Build history of the part. All positions in model axes, mm. Give positions to 0.01 mm unless a question says otherwise; leave off trailing zeros. Write each loop counter-clockwise with the first axis right and the second up, starting at its lowest first coordinate (ties: lowest second). Pieces come first, ordered by that corner, then holes. Notation, with made-up numbers: (54, -36.5) -> (97, -36.5) arc R29 ccw to (97, -7.5) -> close; hole circle Ø3 at (89, 79.25). An arc over 180 degrees is marked (long way). Put each result on its own line as item: value.
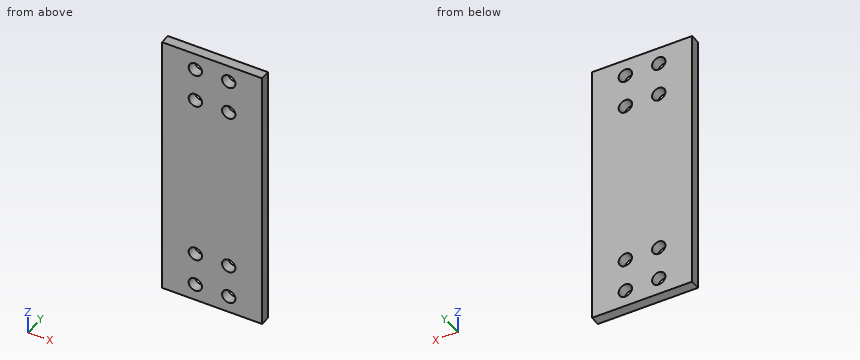
from build123d import *

# Parameters (mm, degrees)
SKETCH2_W           = 15
SKETCH2_H           = 40
SKETCH2_R           = 2
BOSS_EXTRUDE1_DEPTH = 3
MIRROR1_OUTLINE_R   = 2
MIRROR1_DEPTH       = 3


# Read off the part's stored shape, not the designer's step: Mirror1
with BuildPart() as part:
    # Sketch2 → Boss-Extrude1 (new body)
    with BuildSketch(Plane(origin=(0, 0, 0), x_dir=(1, 0, 0), z_dir=(0, 1, 0))):
        with Locations((-7.5, 20)):
            Rectangle(SKETCH2_W, SKETCH2_H)
        with Locations(Location((-5, 35, 0), (0, 0, 270))):
            Circle(SKETCH2_R, mode=Mode.SUBTRACT)
        with Locations(Location((-5, 25, 0), (0, 0, 270))):
            Circle(SKETCH2_R, mode=Mode.SUBTRACT)
    extrude(amount=BOSS_EXTRUDE1_DEPTH)

    # Mirror1 outline → Mirror1 (add)
    with BuildSketch(Plane(origin=(0, 0, 0), x_dir=(1, 0, 0), z_dir=(0, 1, 0))):
        Polygon((15, 40), (0, 40), (0, 0), (-15, 0), (-15, -40), (15, -40), align=None)
        with Locations((-5, -35)):
            Circle(MIRROR1_OUTLINE_R, mode=Mode.SUBTRACT)
        with Locations((-5, -25)):
            Circle(MIRROR1_OUTLINE_R, mode=Mode.SUBTRACT)
        with Locations((5, -35)):
            Circle(MIRROR1_OUTLINE_R, mode=Mode.SUBTRACT)
        with Locations((5, -25)):
            Circle(MIRROR1_OUTLINE_R, mode=Mode.SUBTRACT)
        with Locations((5, 25)):
            Circle(MIRROR1_OUTLINE_R, mode=Mode.SUBTRACT)
        with Locations((5, 35)):
            Circle(MIRROR1_OUTLINE_R, mode=Mode.SUBTRACT)
    extrude(amount=MIRROR1_DEPTH)


solid = part.part
1) Pin check, flat tip, straight feed: pin 1 (2.5 mm diameter, centred on x = 5, z = -25, fed in from +Y). Stop position of the tip, or through.
Filled sheet:
pin 1: through
2) Slice it at C-C (z = -25). Write the cut outline in (x, y), plus the area to 3 significant figures.
Filled sheet:
outline: (-15, 0) -> (-7, 0) -> (-7, 3) -> (-15, 3) -> close; (-3, 0) -> (3, 0) -> (3, 3) -> (-3, 3) -> close; (7, 0) -> (15, 0) -> (15, 3) -> (7, 3) -> close
area: 66.0 mm2
3) Slice it at D-D (x = -6.25). Write the cut outline in (y, z).
Filled sheet:
outline: (0, -40) -> (3, -40) -> (3, -36.56) -> (0, -36.56) -> close; (0, -33.44) -> (3, -33.44) -> (3, -26.56) -> (0, -26.56) -> close; (0, -23.44) -> (3, -23.44) -> (3, 23.44) -> (0, 23.44) -> close; (0, 26.56) -> (3, 26.56) -> (3, 33.44) -> (0, 33.44) -> close; (0, 36.56) -> (3, 36.56) -> (3, 40) -> (0, 40) -> close
4) Slice it at A-A (x = 5). Write the cut outline in (y, z).
Filled sheet:
outline: (0, -40) -> (3, -40) -> (3, -37) -> (0, -37) -> close; (0, -33) -> (3, -33) -> (3, -27) -> (0, -27) -> close; (0, -23) -> (3, -23) -> (3, 23) -> (0, 23) -> close; (0, 27) -> (3, 27) -> (3, 33) -> (0, 33) -> close; (0, 37) -> (3, 37) -> (3, 40) -> (0, 40) -> close
5) Slice it at B-B (y = 2.3). Give the number of separate pieces and of enclosed holes in the cut face, plus the area to 3 significant figures.
Filled sheet:
separate pieces: 1
enclosed holes: 8
area: 2,300 mm2
6) Wall check: L1, parallel to Z at x = 5, y = 0.7; L2, parallel to X at y = 1.9, z = 35; L3, parallel to X at y = 1.15, z = -23.5. Give the ranges that are in metal, low to high.
Filled sheet:
L1: -40 to -37, -33 to -27, -23 to 23, 27 to 33, 37 to 40
L2: -15 to -7, -3 to 3, 7 to 15
L3: -15 to -6.32, -3.68 to 3.68, 6.32 to 15
